Geometry check sheet. Reference: the model listing, model coordinates, mm. Face numbers are marked on the shaded views. Round coordinates to 2 decimals unless told otherwise and drop trailing zeros. Loops run counter-clockwise (first coordinate to the right, second up) from the corner with the lowest first, then second, coordinate; pieces in that order, holes last. Notation, with made-up numbers: (-24, 13) - (14, 13) arc R14 cw to (14, 22) - close; hole circle Ø1 at (-17, 51.25). An arc over 180 degrees is marked (long way). Answer as CSV lines item,"result". Start each with the question number.
1) Thickness scan on line 1 along Y through (x, z) = (0, 1); line 2 along Z through (x, y) = (0.25, 71); line 3 along Y through (x, z) = (0, -4.5). Record the ranges inside material, lowest first.
2) Cross-section at B-B on x = 0. Record the boundary of the cut face in (y, z), and give its area (3 significant figures).
3) Cross-section at C-C on y = 68. Record the boundary of the cut face in (x, z).
4) Cross-section at D-D on y = 46.5. Record the boundary of the cut face in (x, z).
5) Draft check along Z on the marked faces 1, 2 and 3. Enter one of: released by +Z, released by -Z, zero draft, split by the parting line, or undercut.
6) Depth check by flat-ended pin: P1, Ø6, axis at x = -4, y = 61, coming from the +Z side; P2, Ø5, axis at x = 3, y = 16, coming from the +Z side; P3, Ø6, axis at y = 59.5, z = -4.5, coming from the -X side. Enter the tip coordinate at first touch or a pass-through.
7) Cross-section at A-A on z = 0. Record the boundary of the cut face in (x, y), and give its area (3 significant figures).
Autodesk Inventor part; units mm, degrees
ref_plane "Work Plane1" through (0, 0, -7.5004) normal (0, 0, -1) x (-1, 0, 0)
ref_plane "YZ Plane" through (0, 0, 0) normal (1, 0, 0) x (0, 1, 0)
ref_plane "XZ Plane" through (0, 0, 0) normal (0, 1, 0) x (-1, 0, 0)
sketch "Sketch1" plane through (0, 0, 0) normal (0, 1, 0) x (-1, 0, 0)
  circle A0 centre (0, 0) radius 7.5004
extrude "Extrusion1" add sketch "Sketch1" along normal blind 80
sketch "Sketch2" plane through (0, 80, 0) normal (0, 1, 0) x (1, 0, 0)
  point P0 (0, 0)
hole "Hole1" at (0, 80, 0) direction (0, -1, 0) diameter 8.8 depth 30
thread "Thread1"
hole "Hole2" at (0, 0, 0) direction (0, 1, 0) diameter 8.8 depth 30
sketch "Sketch6" plane through (0, 0, 0) normal (1, 0, 0) x (0, 1, 0)
  line L0 (0, -7.5004) -> (0, 7.5004)
  line L1 (0, -7.5004) -> (40, -7.5004)
  line L2 (0, -7.5004) -> (80, -7.5004)
  point P0 (0, 0)
ref_plane "Work Plane1" through (0, 0, -7.5004) normal (0, 0, -1) x (-1, 0, 0)
sketch "Sketch7" plane through (0, 0, -7.5004) normal (0, 0, -1) x (-1, 0, 0)
  line L0 (0, 0) -> (0, 40)
  circle A0 centre (0, 40) radius 4.4
  dimension "d22" = 40
  dimension "d23" = 8.8
hole "Hole3" at (0, 40, -7.5004) direction (0, 0, 1) diameter 9 end through all
thread "Thread3"
thread "Thread4"
fillet "Fillet1" radius 2 2 edges at (7.5004, 0, 0) (7.5004, 80, 0)
properties part number "_3DPrint"
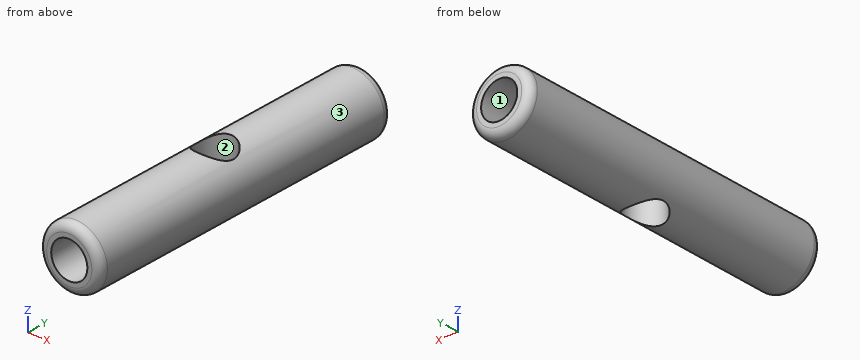
Answer block:
1,line 1,"y = 30 to 35.5, 44.5 to 50"
1,line 2,"z = -7.5 to -4.39, 4.39 to 7.5"
1,line 3,"y = 0 to 35.5, 44.5 to 80"
2,outline,"(0, -5.5) arc R2 ccw to (2, -7.5) - (35.5, -7.5) - (35.5, 7.5) - (2, 7.5) arc R2 ccw to (0, 5.5) - (0, 4.4) - (30, 4.4) - (30, -4.4) - (0, -4.4) - close; (44.5, -7.5) - (78, -7.5) arc R2 ccw to (80, -5.5) - (80, -4.4) - (50, -4.4) - (50, 4.4) - (80, 4.4) - (80, 5.5) arc R2 ccw to (78, 7.5) - (44.5, 7.5) - close"
2,area,"534 mm^2"
3,outline,"circle Ø15 at (0, 0); hole circle Ø8.8 at (0, 0)"
4,outline,"circle Ø15 at (0, 0)"
5,face 1,"undercut"
5,face 2,"zero draft"
5,face 3,"split by the parting line"
6,P1,"stops at z = 7.43"
6,P2,"stops at z = 7.48"
6,P3,"stops at x = -7.35"
7,outline,"(-7.5, 2) arc R2 ccw to (-5.5, 0) - (-4.4, 0) - (-4.4, 30) - (4.4, 30) - (4.4, 0) - (5.5, 0) arc R2 ccw to (7.5, 2) - (7.5, 78) arc R2 ccw to (5.5, 80) - (4.4, 80) - (4.4, 50) - (-4.4, 50) - (-4.4, 80) - (-5.5, 80) arc R2 ccw to (-7.5, 78) - close; hole circle Ø9 at (0, 40)"
7,area,"605 mm^2"
